Here's how the part is built. I have some questions about the finished solid (model axes, mm). Face numbers are marked on the shaded views. A direction names the side the tool comes from. Round coordinates to 2 decimals unless told otherwise and drop trailing zeros. Order: outer loops, then holes, each group sorted by start corner. A loop starts at its lowest first (then second) coordinate and runs counter-clockwise, first axis right, second up.
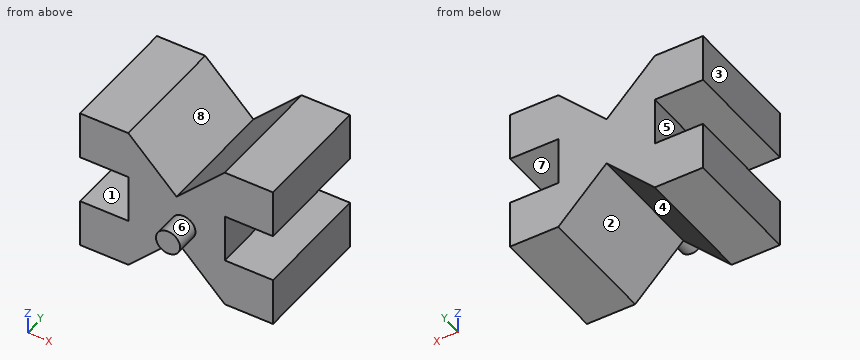
```python
from build123d import *

# Parameters (mm, degrees)
F1_DEPTH = 25
F3_R     = 2.5
F4_DEPTH = 5


with BuildPart() as f1:
    # F0 (on Front) → F1 (new body)
    with BuildSketch(Plane.XZ):
        Polygon((-10, 5), (-10, 0), (-10, -5), (-20, -5), (-20, -15), (-10, -15), (0, -5), (10, -15), (20, -15), (20, -5), (10, -5), (10, 0), (10, 5), (20, 5), (20, 15), (10, 15), (0, 5), (-10, 15), (-20, 15), (-20, 5), align=None)
    extrude(amount=F1_DEPTH)

    # F3 (on face) → F4 (join)
    with BuildSketch(Plane.XZ.offset(25)):
        with Locations((1.424529, -1.24434)):
            Circle(F3_R)
    extrude(amount=F4_DEPTH)


solid = f1.part
```
1) I'm going to push flat-ended pins straight in: pin 1 (8 mm diameter, centred on x = -1.5, z = 7, fed in from -Y); pin 2 (4 mm diameter, centred on x = 3, y = -5, fed in from -Z); pin 3 (1.5 mm diameter, centred on y = -24.5, z = 4, fed in from -X). Where does each tip first touch, or does it pass through?
2) If we section it at D-D (x = 6.5): Write out the boundary of the cut face in (y, z).
3) If we section it at C-C (y = -11): Write out the boundary of the cut face in (x, z), plus the area to 3 significant figures.
4) If we section it at A-A (z = -8): Write out the boundary of the cut face in (x, y), plus the area to 3 significant figures.
5) If we section it at B-B (x = -13.5): Write out the boundary of the cut face in (y, z), plus the area to 3 significant figures.
6) I need wall thicknesses on line 1 (Z direction, x = 11, y = -8); line 2 (Y direction, x = 9, z = -2); line 3 (X direction, y = -21, z = -7.5). Which ranges of each line are inside material? Lowest first, please.
7) We'd pull the mould along X, two halves only. Please class the marked faces 1, 2, 3 and 4: +X half, -X half, draft (parallel to the pull), parting line (faces both ways), or undercut.
8) For the marked faces 5, 6, 7 and 8, which set-ups out of +Z, -Z, +X, -X, +Y, -Y let a thin tool reach every point of the face, with its end or its side?
Solutions:
1. pin 1: stops at y = -25
1. pin 2: stops at z = -10
1. pin 3: stops at x = -10
2. outline: (-25, -11.5) - (0, -11.5) - (0, 11.5) - (-25, 11.5) - close
3. outline: (-20, -15) - (-10, -15) - (0, -5) - (10, -15) - (20, -15) - (20, -5) - (10, -5) - (10, 5) - (20, 5) - (20, 15) - (10, 15) - (0, 5) - (-10, 15) - (-20, 15) - (-20, 5) - (-10, 5) - (-10, -5) - (-20, -5) - close
3. area: 800 mm2
4. outline: (-20, -25) - (-3, -25) - (-3, 0) - (-20, 0) - close; (3, -25) - (20, -25) - (20, 0) - (3, 0) - close
4. area: 850 mm2
5. outline: (-25, -15) - (0, -15) - (0, -5) - (-25, -5) - close; (-25, 5) - (0, 5) - (0, 15) - (-25, 15) - close
5. area: 500 mm2
6. line 1: z = -15 to -5, 5 to 15
6. line 2: y = -25 to 0
6. line 3: x = -20 to -2.5, 2.5 to 20
7. face 1: draft
7. face 2: undercut
7. face 3: -X half
7. face 4: undercut
8. face 5: -X, +Y, -Y
8. face 6: -Y
8. face 7: +X, +Y, -Y
8. face 8: +Z, +Y, -Y
